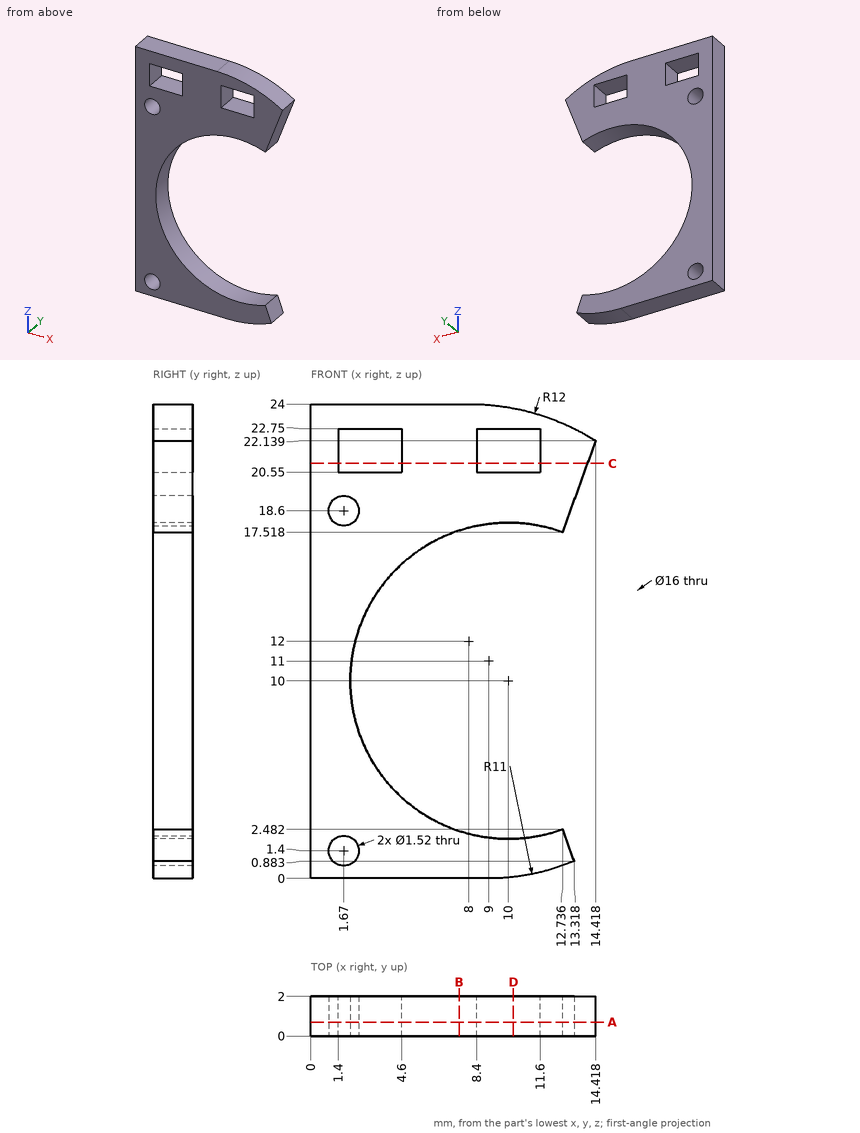
Here's the drawing with two shaded views (mm, measured from the low corner). I have some questions. Coordinates: 2 decimals unless noted, no trailing zeros. Loops run counter-clockwise (first coordinate to the right, second up) from the corner with the lowest first, then second, coordinate; pieces in that order, holes last. Notation, with made-up numbers: M 39,-21 L 75,-21 A24 ccw 75,9 Z; hole C 29.5,-16 d4. An arc over 180 degrees is marked long. Answer as CSV lines item,"result". Start each with the question number.
1. If I drill on probe 1 along X at (y, z) = (0.8, 20.75); probe 2 along Z at (x, y) = (7.25, 0.5); probe 3 along X at (y, z) = (1.5, 10), over which ranges is the centre line in solid material (lowest first)? Write a range as [from, to].
2. For pin 1 Ø1 at (x, y) = (10, 1) entering from +Z; pin 2 Ø0.6 at (y, z) = (1.5, 21.5) entering from +X (1 decimal); pin 3 Ø2 at (x, z) = (6.5, 16.5) entering from -Y; pin 4 Ø1 at (x, z) = (9.5, 16) entering from -Y, each with a flat end and sliding along its axis, tell me the tip position at first contact or that it passes through.
3. Suppose I cut it at C-C, the plane z = 21. List the corners of the cut face in (x, y) for me.
4. Suppose I cut it at D-D, the plane x = 10.25. List the corners of the cut face in (y, z) for me.
5. Suppose I cut it at A-A, the plane y = 0.7. List the corners of the cut face in (x, z) for me.
6. Suppose I cut it at B-B, the plane x = 7.5. List the corners of the cut face in (y, z) for me, plus the area to 3 significant figures.
Output:
1,probe 1,"x = [0, 1.4], [4.6, 8.4], [11.6, 13.91]"
1,probe 2,"z = [0, 2.49], [17.51, 24]"
1,probe 3,"x = [0, 2]"
2,pin 1,"stops at z = 23.91"
2,pin 2,"stops at x = 14.3"
2,pin 3,"stops at y = 0"
2,pin 4,"passes through"
3,outline,"M 0,0 L 1.4,0 L 1.4,2 L 0,2 Z; M 4.6,0 L 8.4,0 L 8.4,2 L 4.6,2 Z; M 11.6,0 L 14,0 L 14,2 L 11.6,2 Z"
4,outline,"M 0,0.07 L 2,0.07 L 2,2 L 0,2 Z; M 0,18 L 2,18 L 2,20.55 L 0,20.55 Z; M 0,22.75 L 2,22.75 L 2,23.79 L 0,23.79 Z"
5,outline,"M 0,0 L 9,0 A11 ccw 13.32,0.88 L 12.74,2.48 A8 cw long 12.74,17.52 L 14.42,22.14 A12 ccw 8,24 L 0,24 Z; hole C 1.67,1.4 d1.52; hole C 1.67,18.6 d1.52; hole M 1.4,20.55 L 4.6,20.55 L 4.6,22.75 L 1.4,22.75 Z; hole M 8.4,20.55 L 11.6,20.55 L 11.6,22.75 L 8.4,22.75 Z"
6,outline,"M 0,0 L 2,0 L 2,2.4 L 0,2.4 Z; M 0,17.6 L 2,17.6 L 2,24 L 0,24 Z"
6,area,"17.6 mm^2"
